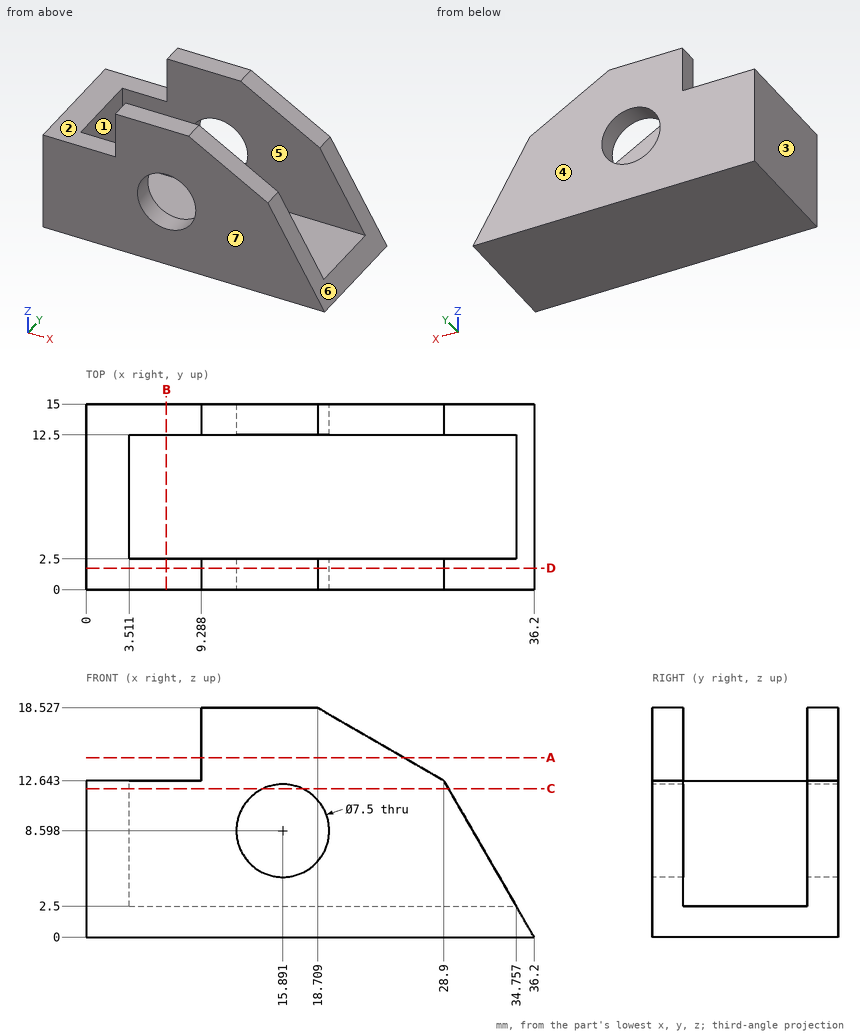
Verification items for this drawing (mm, ordinates from the low corner). A direction names the side the tool comes from. Give positions to 0.01 mm unless a question says otherwise; leave off trailing zeros. Write each loop counter-clockwise with the first axis right and the second up, starting at its lowest first coordinate (ties: lowest second). Pieces come first, ordered by that corner, then holes.
1) Cross-section at A-A (z = 14.5). Record the boundary of the cut face in (x, y) (1 decimal).
Values follow:
outline: (9.3, 0) - (25.7, 0) - (25.7, 2.5) - (9.3, 2.5) - close; (9.3, 12.5) - (25.7, 12.5) - (25.7, 15) - (9.3, 15) - close
2) Go/stop test with flat-tipped pins: pin 1 Ø0.8 at (y, z) = (1, 15.5) entering from -X; pin 2 Ø3 at (x, y) = (29, 8.5) entering from +Z; pin 3 Ø6 at (y, z) = (6, 2.5) entering from +X; pin 4 Ø7 at (x, z) = (15.89, 8.6) entering from -Y. Record where each tip stops, or that it passes through.
Values follow:
pin 1: stops at x = 9.29
pin 2: stops at z = 2.5
pin 3: stops at x = 36.2
pin 4: passes through
3) Cross-section at C-C (z = 12). Record the boundary of the cut face in (x, y) (1 decimal), plus the area to 3 significant figures.
Values follow:
outline: (0, 0) - (14.3, 0) - (14.3, 2.5) - (3.5, 2.5) - (3.5, 12.5) - (14.3, 12.5) - (14.3, 15) - (0, 15) - close; (17.5, 0) - (29.3, 0) - (29.3, 2.5) - (17.5, 2.5) - close; (17.5, 12.5) - (29.3, 12.5) - (29.3, 15) - (17.5, 15) - close
area: 166 mm2
4) Set-up check for the marked faces 1, 2 and 3: record each of +Z, -Z, +X, -X, +Y, -Y from which the full face is reachable in a straight line by a thin tool's end or side.
Values follow:
face 1: +Z, +X
face 2: +Z, -X, +Y, -Y
face 3: +Z, -Z, -X, +Y, -Y
5) Thickness scan on line 1 (Y direction, x = 33, z = 5); line 2 (Z direction, x = 7.5, y = 8); line 3 (X direction, y = 2.75, z = 12). Record the ranges inside material, lowest first.
Values follow:
line 1: y = 0 to 2.5, 12.5 to 15
line 2: z = 0 to 2.5
line 3: x = 0 to 3.51
6) Cross-section at B-B (x = 6.5). Record the boundary of the cut face in (y, z).
Values follow:
outline: (0, 0) - (15, 0) - (15, 12.64) - (12.5, 12.64) - (12.5, 2.5) - (2.5, 2.5) - (2.5, 12.64) - (0, 12.64) - close
7) Cross-section at D-D (y = 1.75). Record the boundary of the cut face in (x, z).
Values follow:
outline: (0, 0) - (36.2, 0) - (28.9, 12.64) - (18.71, 18.53) - (9.29, 18.53) - (9.29, 12.64) - (0, 12.64) - close; hole circle Ø7.5 at (15.89, 8.6)
8) Release check for a two-part mould opening along Y. For the marked faces 4, 5, 6 and 7 record: released by +Y, released by -Y, zero draft, split by the parting line, or undercut.
Values follow:
face 4: released by +Y
face 5: undercut
face 6: zero draft
face 7: released by -Y
